Verification items for the finished model (mm, model axes). Coordinates: 2 decimals unless noted, no trailing zeros. Loops run counter-clockwise (first coordinate to the right, second up) from the corner with the lowest first, then second, coordinate; pieces in that order, holes last. Notation, with made-up numbers: (68.5, 55) -> (81.5, 55) arc R24 cw to (81.5, 76) -> close; hole circle Ø2 at (16.5, 56.25). An arc over 180 degrees is marked (long way). Write item = value, one per line.
```python
from build123d import *

# Parameters (mm, degrees)
SKETCH_R     = 3.25
PAD_DEPTH    = 10
SKETCH001_R  = 4
PAD001_DEPTH = 10
SKETCH002_R  = 3
PAD002_DEPTH = 6
PAD003_DEPTH = 4


with BuildPart() as part:
    # Sketch → Pad (new body)
    with BuildSketch(Plane.XY):
        Circle(SKETCH_R)
    extrude(amount=PAD_DEPTH)

    # Sketch001 → Pad001 (join)
    with BuildSketch(Plane(origin=(0, 0, 0), x_dir=(1, 0, 0), z_dir=(0, -0.707107, -0.707107))):
        Circle(SKETCH001_R)
    extrude(amount=PAD001_DEPTH)

    # Sphere → Sphere (revolve)
    with BuildSketch(Plane.XZ):
        with BuildLine():
            ThreePointArc((0, -4), (4, 0), (0, 4))
            Line((0, 4), (0, -4))
        make_face()
    revolve(axis=Axis((0, 0, 0), (0, 0, 1)))

    # Sphere001 → Sphere001 (revolve)
    with BuildSketch(Plane(origin=(0, 0, 10), x_dir=(1, 0, 0), z_dir=(0, 0, -1))):
        with BuildLine():
            ThreePointArc((0, -4), (4, 0), (0, 4))
            Line((0, 4), (0, -4))
        make_face()
    revolve(axis=Axis((0, 0, 10), (0, -1, 0)))

    # Sketch002 (on Face6 of Sphere001) → Pad002 (join)
    with BuildSketch(Plane(origin=(0, -12.071068, -2.071068), x_dir=(1, 0, 0), z_dir=(0, -0.707107, -0.707107))):
        with Locations((0, -7.071068)):
            Circle(SKETCH002_R)
    extrude(amount=PAD002_DEPTH)

    # Sketch003 (on Face6 of Pad002) → Pad003 (join)
    with BuildSketch(Plane(origin=(0, -12.071068, -2.071068), x_dir=(1, 0, 0), z_dir=(0, -0.707107, -0.707107))):
        Polygon((2.367136, -2.971068), (-2.367136, -2.971068), (-4.734272, -7.071068), (-2.367136, -11.171068), (2.367136, -11.171068), (4.734272, -7.071068), align=None)
    extrude(amount=-PAD003_DEPTH)


solid = part.part
```
1) Release check for a two-part mould opening along Z. For faces 1 (the face through (3.534, -4.207, -7.147)), 2 (the face through (0, -8.6, -2.8)), 3 (the face through (4.186, -4.256, -4.229)), 4 (the face through (-2.579, -1.978, 4.963)) record: pulls with the +Z half, pulls with the -Z half, needs draft (parallel to the pull), parting line crosses it, or undercut.
Ans:
face_1 = pulls with the -Z half
face_2 = pulls with the +Z half
face_3 = undercut
face_4 = undercut
2) Sectioned sample at B-B, the plane z = 2.75. Record the cut outline in (x, y), plus the area to 3 significant figures.
Ans:
outline = circle Ø6.5 at (0, 0)
area = 33.2 mm2
3) Material ranges on line 1 (Y direction, x = -1.25, z = 2.5); line 2 (X direction, y = 1.75, z = 4.75); line 3 (Y direction, x = -3, z = 1.75), recorded low to high.
Ans:
line_1 = -3 to 3
line_2 = -2.74 to 2.74
line_3 = -1.99 to 1.98
4) Sectioned sample at A-A, the plane x = 0. Record the cut outline in (y, z).
Ans:
outline = (-13.44, -9.19) -> (-9.19, -13.44) -> (-4.95, -9.19) -> (-4.17, -9.97) -> (-1.34, -7.14) -> (-1.41, -7.07) -> (2.83, -2.83) arc R4 ccw to (3.25, 2.33) -> (3.25, 7.67) arc R4 ccw (long way) to (-3.25, 7.67) -> (-3.25, 2.41) -> (-7.07, -1.41) -> (-7.14, -1.34) -> (-9.97, -4.17) -> (-9.19, -4.95) -> close
5) Depth check by flat-ended pin: pin 1 Ø1 at (x, z) = (1.5, 5.5) entering from -Y; pin 2 Ø6 at (y, z) = (-4, 6.5) entering from +X; pin 3 Ø8 at (y, z) = (-6, 11) entering from -X (3 decimals). Enter the tip coordinate at first touch or a pass-through.
Ans:
pin_1 = -3.09
pin_2 = 3.26
pin_3 = -3.415
